Part model, mm, in its own coordinate system. A direction names the side the tool comes from. Round coordinates to 2 decimals unless told otherwise and drop trailing zeros. Order: outer loops, then holes, each group sorted by start corner. A loop starts at its lowest first (then second) coordinate and runs counter-clockwise, first axis right, second up. Notation, with made-up numbers: M 51,64 L 61,64 A21 ccw 61,72 Z; hole C -33,-22 d9. An arc over 180 degrees is marked long. One line per question, with ' | ' between items.
from build123d import *

# Parameters (mm, degrees)
F0_W     = 101.5
F0_H     = 48
F1_DEPTH = 1.8
F2_W     = 101.5
F2_H     = 1.8
F3_DEPTH = 16
F4_DEPTH = 32
F5_R     = 2
F6_R     = 2.4
F6_R_2   = 2
F7_DEPTH = 48.001


with BuildPart() as f1:
    # F0 (on Front) → F1 (new body)
    with BuildSketch(Plane.XZ):
        with Locations((50.75, 24)):
            Rectangle(F0_W, F0_H)
    extrude(amount=F1_DEPTH)

    # F2 (on face) → F3 (join)
    with BuildSketch(Plane.XZ.offset(1.8)):
        with Locations((50.75, 0.9)):
            Rectangle(F2_W, F2_H)
    extrude(amount=F3_DEPTH)

    # F2 (on face) → F4 (join)
    with BuildSketch(Plane.XZ.offset(1.8)):
        with Locations((50.75, 47.1)):
            Rectangle(F2_W, F2_H)
    extrude(amount=-F4_DEPTH)

    # F5
    f5_edges = [f1.edges().sort_by_distance(p)[0] for p in [
        (50.75, -1.8, 48),
        (50.75, -1.8, 1.8),
        (50.75, 0, 46.2),
        (50.75, 0, 0),
    ]]
    fillet(f5_edges, radius=F5_R)

    # F6 (on face) → F7 (cut, through all)
    with BuildSketch(Plane.XY.offset(48)):
        with Locations((15.8, 16)):
            Circle(F6_R)
        with Locations((21.75, 23.95)):
            Circle(F6_R_2)
        with BuildLine():
            ThreePointArc((17.5665768757, 24.8), (15.5665768757, 26.8), (13.5665768757, 24.8))
            Line((13.5665768757, 24.8), (13.5665768757, 23.8))
            ThreePointArc((13.5665768757, 23.8), (15.5665768757, 21.8), (17.5665768757, 23.8))
            Line((17.5665768757, 23.8), (17.5665768757, 24.8))
        make_face()
        with Locations((32.9, 14)):
            Circle(F6_R_2)
        with BuildLine():
            Line((87.9334231243, 23.8), (87.9334231243, 24.8))
            ThreePointArc((87.9334231243, 24.8), (85.9334231243, 26.8), (83.9334231243, 24.8))
            Line((83.9334231243, 24.8), (83.9334231243, 23.8))
            ThreePointArc((83.9334231243, 23.8), (85.9334231243, 21.8), (87.9334231243, 23.8))
        make_face()
        with Locations((79.75, 23.95)):
            Circle(F6_R_2)
        with Locations((85.7, 16)):
            Circle(F6_R)
        with Locations((68.6, 14)):
            Circle(F6_R_2)
        with BuildLine():
            Line((53.1334231243, 23.8), (53.1334231243, 24.8))
            ThreePointArc((53.1334231243, 24.8), (51.1334231243, 26.8), (49.1334231243, 24.8))
            Line((49.1334231243, 24.8), (49.1334231243, 23.8))
            ThreePointArc((49.1334231243, 23.8), (51.1334231243, 21.8), (53.1334231243, 23.8))
        make_face()
        with Locations((51.3668462485, 16)):
            Circle(F6_R)
        with BuildLine():
            Line((37.6, 30.2), (28.8, 30.2))
            Line((28.8, 30.2), (28.8, 23.2))
            ThreePointArc((28.8, 23.2), (33.2, 18.8), (37.6, 23.2))
            Line((37.6, 23.2), (37.6, 30.2))
        make_face()
        with BuildLine():
            Line((72.7, 30.2), (63.9, 30.2))
            Line((63.9, 30.2), (63.9, 23.2))
            ThreePointArc((63.9, 23.2), (68.3, 18.8), (72.7, 23.2))
            Line((72.7, 23.2), (72.7, 30.2))
        make_face()
    extrude(amount=-F7_DEPTH, mode=Mode.SUBTRACT)


solid = f1.part
1) Saw through at A-A (x = 21.75). List the corners of the cut face in (y, z), plus the area to 3 significant figures.
The answers:
outline: M -17.8,0 L -2,0 A2 ccw 0,2 L 0,44.2 A2 cw 2,46.2 L 21.95,46.2 L 21.95,48 L 0.2,48 A2 ccw -1.8,46 L -1.8,3.8 A2 cw -3.8,1.8 L -17.8,1.8 Z; M 25.95,46.2 L 30.2,46.2 L 30.2,48 L 25.95,48 Z | area: 162 mm²
2) Probe line 1 (Z direction, x = 53.5, y = -6); line 2 (Y direction, x = 32, z = 47); line 3 (Z direction, x = 6, y = 19.5). List the from-to ranges inside material, lowest first. Write a range as [from, to].
The answers:
line 1: z = [0, 1.8] | line 2: y = [-1.53, 12.21], [15.79, 18.97] | line 3: z = [46.2, 48]
3) Saw through at B-B (x = 76.5). List the corners of the cut face in (y, z), plus the area to 3 significant figures.
The answers:
outline: M -17.8,0 L -2,0 A2 ccw 0,2 L 0,44.2 A2 cw 2,46.2 L 30.2,46.2 L 30.2,48 L 0.2,48 A2 ccw -1.8,46 L -1.8,3.8 A2 cw -3.8,1.8 L -17.8,1.8 Z | area: 170 mm²
4) Saw through at C-C (z = 33.5). List the corners of the cut face in (x, y).
The answers:
outline: M 0,-1.8 L 101.5,-1.8 L 101.5,0 L 0,0 Z
5) Two-plate mould, pull along X, no slides. Class faces 5 (the face through (0, -1, 27)), 6 (the face through (51.46, -2.37, 2.4)), 7 (the face through (13.402, 16.106, 47.113)), 8 (the face through (85.9, 21.8, 47.1)): released by +X, released by -X, zero draft, split by the parting line, or undercut.
The answers:
face 5: released by -X | face 6: zero draft | face 7: undercut | face 8: undercut
6) Drop flat-ended pins along their axis: pin 1 (4.5 mm diameter, centred on x = 68.6, y = 14, fed in from +Z); pin 2 (6 mm diameter, centred on x = 89, z = 24, fed in from -Y); pin 3 (7 mm diameter, centred on x = 52, y = -10.5, fed in from +Z); pin 4 (10 mm diameter, centred on x = 68, z = 29, fed in from +Y). Give the stop position or say it passes through.
The answers:
pin 1: stops at z = 48 | pin 2: stops at y = -1.8 | pin 3: stops at z = 1.8 | pin 4: stops at y = 0
7) Which spindle directions (+Z, -Z, +X, -X, +Y, -Y) get a long thin tool onto all of the face, cutting with end or side? Do faces 1 (the face through (68.2, 18.8, 47.1)), 2 (the face through (50, 13, 46.2)), 3 (the face through (50, -11, 1.8)), 4 (the face through (15.6, 26.8, 47.1)). Say none if no direction does.
The answers:
face 1: +Z, -Z, +Y | face 2: -Z, +X, -X, +Y | face 3: +Z, +X, -X, -Y | face 4: +Z, -Z
8) Saw through at D-D (y = -6.5). List the corners of the cut face in (x, z), plus the area to 3 significant figures.
The answers:
outline: M 0,0 L 101.5,0 L 101.5,1.8 L 0,1.8 Z | area: 183 mm²
